Verification items for the finished model (mm, model axes). Give positions to 0.01 mm unless a question says otherwise; leave off trailing zeros. Loops run counter-clockwise (first coordinate to the right, second up) from the corner with the lowest first, then second, coordinate; pieces in that order, holes last. Notation, with made-up numbers: M 48,57.5 L 78,57.5 A28 ccw 78,93.5 Z; hole C -21.5,-28.75 d9. An arc over 180 degrees is marked long. Use a Markdown table: item, result.
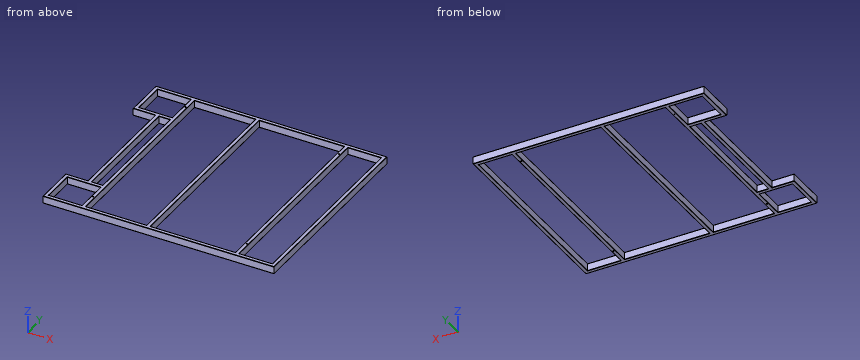
from build123d import *

# Parameters (mm, degrees)
F0_W     = 228.6
F0_H     = 228.6
F0_W_2   = 76.2
F0_H_2   = 825.5
F0_W_3   = 419.1
F0_H_3   = 1333.5
F0_W_4   = 584.2
F1_DEPTH = 25.4
F2_R     = 2.3622
F3_R     = 2.3622
F5_D     = 8.73125


with BuildPart() as f1:
    # F0 (on Top) → F1 (new body, symmetric)
    with BuildSketch(Plane.XY):
        Polygon((-927.9385305348, -419.3321948051), (-927.9385305348, -698.7321948051), (659.5614694652, -698.7321948051), (659.5614694652, 685.5678051949), (-927.9385305348, 685.5678051949), (-927.9385305348, 406.1678051949), (-775.5385305348, 406.1678051949), (-775.5385305348, -419.3321948051), align=None)
        with Locations((-788.2385305348, -559.0321948051)):
            Rectangle(F0_W, F0_H, mode=Mode.SUBTRACT)
        with Locations((-712.0385305348, -6.5821948051)):
            Rectangle(F0_W_2, F0_H_2, mode=Mode.SUBTRACT)
        with Locations((-438.9885305348, -6.5821948051)):
            Rectangle(F0_W_3, F0_H_3, mode=Mode.SUBTRACT)
        with Locations((-788.2385305348, 545.8678051949)):
            Rectangle(F0_W, F0_H, mode=Mode.SUBTRACT)
        with Locations((88.0614694652, -6.5821948051)):
            Rectangle(F0_W_4, F0_H_3, mode=Mode.SUBTRACT)
        with Locations((519.8614694652, -6.5821948051)):
            Rectangle(F0_W, F0_H_3, mode=Mode.SUBTRACT)
    extrude(amount=F1_DEPTH, both=True)

    # F2
    f2_edges = [f1.edges().sort_by_distance(p)[0] for p in [
        (-927.938531, 545.867805, 25.4),
        (-851.738531, 406.167805, 25.4),
        (-775.538531, -6.582195, 25.4),
        (-134.188531, 685.567805, 25.4),
        (659.561469, -6.582195, 25.4),
        (-134.188531, -698.732195, 25.4),
        (-927.938531, -559.032195, 25.4),
        (-851.738531, -419.332195, 25.4),
        (-712.038531, -419.332195, 25.4),
        (-750.138531, -6.582195, 25.4),
        (-788.238531, -444.732195, 25.4),
        (-673.938531, -559.032195, 25.4),
        (-902.538531, -559.032195, 25.4),
        (-788.238531, -673.332195, 25.4),
        (-438.988531, -673.332195, 25.4),
        (-648.538531, -6.582195, 25.4),
        (-229.438531, -6.582195, 25.4),
        (88.061469, -673.332195, 25.4),
        (380.161469, -6.582195, 25.4),
        (519.861469, -673.332195, 25.4),
        (634.161469, -6.582195, 25.4),
        (-204.038531, -6.582195, 25.4),
        (405.561469, -6.582195, 25.4),
        (-902.538531, 545.867805, 25.4),
        (-788.238531, 431.567805, 25.4),
        (-788.238531, 660.167805, 25.4),
        (-438.988531, 660.167805, 25.4),
        (-712.038531, 406.167805, 25.4),
        (-673.938531, -6.582195, 25.4),
        (-673.938531, 545.867805, 25.4),
        (88.061469, 660.167805, 25.4),
        (519.861469, 660.167805, 25.4),
    ]]
    fillet(f2_edges, radius=F2_R)

    # F3
    f3_edges = [f1.edges().sort_by_distance(p)[0] for p in [
        (-927.938531, -559.032195, -25.4),
        (-851.738531, -419.332195, -25.4),
        (-902.538531, -559.032195, -25.4),
        (-673.938531, -559.032195, -25.4),
        (-788.238531, -673.332195, -25.4),
        (-134.188531, -698.732195, -25.4),
        (-438.988531, -673.332195, -25.4),
        (-648.538531, -6.582195, -25.4),
        (-229.438531, -6.582195, -25.4),
        (-204.038531, -6.582195, -25.4),
        (-788.238531, -444.732195, -25.4),
        (88.061469, -673.332195, -25.4),
        (380.161469, -6.582195, -25.4),
        (405.561469, -6.582195, -25.4),
        (519.861469, -673.332195, -25.4),
        (634.161469, -6.582195, -25.4),
        (519.861469, 660.167805, -25.4),
        (88.061469, 660.167805, -25.4),
        (-438.988531, 660.167805, -25.4),
        (-788.238531, 660.167805, -25.4),
        (-927.938531, 545.867805, -25.4),
        (-851.738531, 406.167805, -25.4),
        (-788.238531, 431.567805, -25.4),
        (-673.938531, 545.867805, -25.4),
        (-673.938531, -6.582195, -25.4),
        (-775.538531, -6.582195, -25.4),
        (-750.138531, -6.582195, -25.4),
        (659.561469, -6.582195, -25.4),
        (-712.038531, -419.332195, -25.4),
        (-134.188531, 685.567805, -25.4),
    ]]
    fillet(f3_edges, radius=F3_R)

    # F5 (through all)
    with Locations(Plane(origin=(0, 0, -25.4), x_dir=(1, 0, 0), z_dir=(0, 0, -1))):
        with Locations((-661.2385305348, -571.2678051949), (-661.2385305348, 559.0321948051), (392.8614694652, 559.0321948051), (392.8614694652, -571.2678051949)):
            Hole(F5_D / 2)


solid = f1.part
(1) Gauge pin test, flat end, axial feed: P1, Ø14, axis at y = 55.5, z = -10, coming from the -X side. Record the tip position at first contact, or that the pin passes through.
Results below:
| item | result |
|---|---|
| P1 | x = -775.54 |
(2) Cross-section at A-A on x = 115.5. Record the cut outline in (y, z), then the cut area to 3 significant figures.
Results below:
| item | result |
|---|---|
| outline | M -698.73,-23.04 A2.36 ccw -696.37,-25.4 L -675.69,-25.4 A2.36 ccw -673.33,-23.04 L -673.33,23.04 A2.36 ccw -675.69,25.4 L -696.37,25.4 A2.36 ccw -698.73,23.04 Z; M 660.17,-23.04 A2.36 ccw 662.53,-25.4 L 683.21,-25.4 A2.36 ccw 685.57,-23.04 L 685.57,23.04 A2.36 ccw 683.21,25.4 L 662.53,25.4 A2.36 ccw 660.17,23.04 Z |
| area | 2,570 mm^2 |
(3) Material ranges on line 1 (X direction, y = -386, z = -23); line 2 (X direction, y = -574.5, z = -15); line 3 (X direction, y = 429, z = -8), recorded low to high.
Results below:
| item | result |
|---|---|
| line 1 | -775.54 to -750.14, -673.94 to -648.54, -229.44 to -204.04, 380.16 to 405.56, 634.16 to 659.56 |
| line 2 | -927.94 to -902.54, -673.94 to -648.54, -229.44 to -204.04, 380.16 to 405.56, 634.16 to 659.56 |
| line 3 | -927.94 to -648.54, -229.44 to -204.04, 380.16 to 405.56, 634.16 to 659.56 |
(4) Cross-section at B-B on x = -705.5. State how many separate pieces and enclosed holes the cut face has, then the cut area to 3 significant figures.
Results below:
| item | result |
|---|---|
| separate pieces | 4 |
| enclosed holes | 0 |
| area | 5,140 mm^2 |
